Part model, mm, in its own coordinate system. Face numbers are marked on the shaded views. A direction names the side the tool comes from. Round coordinates to 2 decimals unless told otherwise and drop trailing zeros. Write each loop counter-clockwise with the first axis right and the second up, starting at its lowest first coordinate (ties: lowest second). Pieces come first, ordered by that corner, then holes.
1) Which spindle directions (+Z, -Z, +X, -X, +Y, -Y) get a long thin tool onto all of the face, cutting with end or side? Do the marked faces 4 and 5. Say none if no direction does.
2) Saw through at D-D on x = -68. Write the cut outline in (y, z), and give its area (3 significant figures).
3) Saw through at A-A on y = 5. Write the cut outline in (x, z).
4) Saw through at C-C on z = 138.5. Write the cut outline in (x, y).
5) Drill centre lines: L1, parallel to X at y = 45, z = 75; L2, parallel to X at y = 21.5, z = 96.5; L3, parallel to Y at x = -10, z = 5.2. Where is each one in solid material? Low to high.
6) Pull direction Y, two halves, no side cores. Call the marked faces 1, 2 and 3: +Y half, -Y half, draft (parallel to the pull), parting line (faces both ways), or undercut.
7) Flat gauge pins, fed straight in: pin 1 (5 mm diameter, centred on x = -165.5, z = 118.5, fed in from -Y); pin 2 (11 mm diameter, centred on x = -10.5, z = 93, fed in from -Y); pin 3 (4 mm diameter, centred on x = -10.5, y = 13, fed in from -Z). Where does each tip first touch, or does it go through?
8) Saw through at B-B on x = -10. Write the cut outline in (y, z).
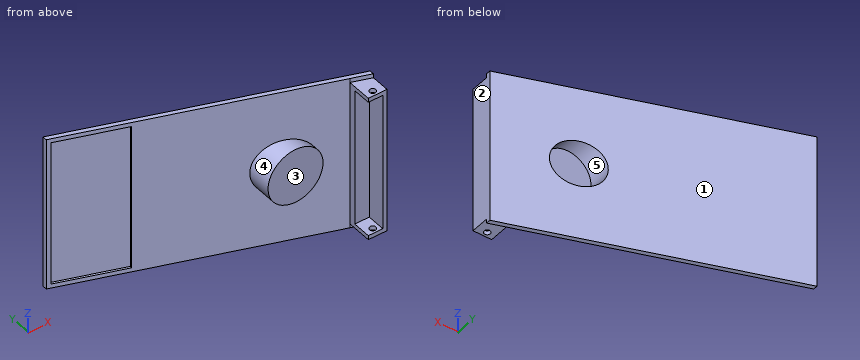
```python
from build123d import *

# Parameters (mm, degrees)
BOSS_EXTRUDE1_DEPTH = 150
CUT_EXTRUDE1_DEPTH  = 4
CUT_EXTRUDE2_DEPTH  = 4
SKETCH4_R           = 3
CUT_EXTRUDE3_DEPTH  = 162
SKETCH6_W           = 134
SKETCH6_H           = 17.5
CUT_EXTRUDE4_DEPTH  = 14
SKETCH9_R           = 22.5
CUT_EXTRUDE5_DEPTH  = 83
SKETCH10_R          = 26.5
BOSS_EXTRUDE2_DEPTH = 55
SKETCH12_R          = 26.5
CUT_EXTRUDE6_DEPTH  = 27
SKETCH13_R          = 22.5
CUT_EXTRUDE7_DEPTH  = 24
SKETCH14_W          = 65
SKETCH14_H          = 142
CUT_EXTRUDE8_DEPTH  = 2
SKETCH15_W          = 73.049040635
SKETCH15_H          = 56.643959476
CUT_EXTRUDE9_DEPTH  = 22


with BuildPart() as part:
    # Sketch1 → Boss-Extrude1 (new body)
    with BuildSketch(Plane.XY):
        Polygon((0, 0), (0, 21.74), (-249.999833435, 109.239715329), (-249.999833435, 104.999731628), (-18, 23.8), (-18, 0), align=None)
    extrude(amount=BOSS_EXTRUDE1_DEPTH)

    # Sketch2 → Cut-Extrude1 (cut)
    with BuildSketch(Plane.XY.offset(150)):
        Polygon((-18, 23.8), (0, 17.500016299), (0, 0), (-18, 0), align=None)
    extrude(amount=-CUT_EXTRUDE1_DEPTH, mode=Mode.SUBTRACT)

    # Sketch3 → Cut-Extrude2 (cut)
    with BuildSketch(Plane(origin=(0, 0, 0), x_dir=(-1, 0, 0), z_dir=(0, 0, -1))):
        Polygon((18, 0), (18, 23.8), (0, 17.500016299), (0, 0), align=None)
    extrude(amount=-CUT_EXTRUDE2_DEPTH, mode=Mode.SUBTRACT)

    # Sketch4 → Cut-Extrude3 (cut)
    with BuildSketch(Plane(origin=(0, 0, 4), x_dir=(-1, 0, 0), z_dir=(0, 0, -1))):
        with Locations((10, 5)):
            Circle(SKETCH4_R)
    extrude(amount=-CUT_EXTRUDE3_DEPTH, mode=Mode.SUBTRACT)

    # Sketch6 → Cut-Extrude4 (cut)
    with BuildSketch(Plane.ZY.offset(18)):
        with Locations((75, 8.75)):
            Rectangle(SKETCH6_W, SKETCH6_H)
    extrude(amount=-CUT_EXTRUDE4_DEPTH, mode=Mode.SUBTRACT)

    # Sketch9 → Cut-Extrude5 (cut)
    with BuildSketch(Plane(origin=(0, 0, 0), x_dir=(1, 0, 0), z_dir=(0, 1, 0))):
        with Locations((-68, -75)):
            Circle(SKETCH9_R)
    extrude(amount=CUT_EXTRUDE5_DEPTH, mode=Mode.SUBTRACT)

    # Sketch10 → Boss-Extrude2 (add)
    with BuildSketch(Plane(origin=(0, 0, 0), x_dir=(1, 0, 0), z_dir=(0, 1, 0))):
        with Locations((-68, -75)):
            Circle(SKETCH10_R)
    extrude(amount=BOSS_EXTRUDE2_DEPTH)

    # Sketch12 → Cut-Extrude6 (cut)
    with BuildSketch(Plane.XZ):
        with Locations(Location((-68, 75, 0), (0, 0, 270))):
            Circle(SKETCH12_R)
    extrude(amount=-CUT_EXTRUDE6_DEPTH, mode=Mode.SUBTRACT)

    # Sketch13 → Cut-Extrude7 (cut)
    with BuildSketch(Plane(origin=(0, 55, 0), x_dir=(1, 0, 0), z_dir=(0, 1, 0))):
        with Locations(Location((-68, -75, 0), (0, 0, 270))):
            Circle(SKETCH13_R)
    extrude(amount=-CUT_EXTRUDE7_DEPTH, mode=Mode.SUBTRACT)

    # Sketch14 → Cut-Extrude8 (cut)
    with BuildSketch(Plane(origin=(5.456564202, 15.590223769, 0), x_dir=(0.9438586228518121, -0.3303496633391366, 0), z_dir=(-0.3303496633391366, -0.9438586228518121, 0))):
        with Locations((-234.151124493, 75)):
            Rectangle(SKETCH14_W, SKETCH14_H)
    extrude(amount=-CUT_EXTRUDE8_DEPTH, mode=Mode.SUBTRACT)

    # Sketch15 → Cut-Extrude9 (cut)
    with BuildSketch(Plane(origin=(6.778605444, 19.367494233, 0), x_dir=(0.9438586228518122, -0.330349663339136, 0), z_dir=(0.330349663339136, 0.9438586228518122, 0))):
        with Locations((-76.286643032, -75.675013618)):
            Rectangle(SKETCH15_W, SKETCH15_H)
    extrude(amount=CUT_EXTRUDE9_DEPTH, mode=Mode.SUBTRACT)


solid = part.part
```
Completed:
1. face 4: -Y
1. face 5: +Y
2. outline: (27, 48.5) - (41.3, 48.5) - (41.3, 0) - (45.54, 0) - (45.54, 52.5) - (31, 52.5) - (31, 97.5) - (45.54, 97.5) - (45.54, 150) - (41.3, 150) - (41.3, 101.5) - (27, 101.5) - close
2. area: 740 mm2
3. outline: (-18, 4) - (-13, 4) - (-13, 8) - (-18, 8) - close; (-18, 142) - (-13, 142) - (-13, 146) - (-18, 146) - close; (-7, 4) - (0, 4) - (0, 146) - (-7, 146) - (-7, 142) - (-4, 142) - (-4, 8) - (-7, 8) - close
4. outline: (-250, 105) - (-246.22, 103.68) - (-245.56, 105.57) - (-184.21, 84.09) - (-184.87, 82.21) - (-18, 23.8) - (-18, 17.5) - (-4, 17.5) - (-4, 0) - (0, 0) - (0, 21.74) - (-250, 109.24) - close
5. L1: x = -94.5 to -90.5
5. L2: x = -18 to 0
5. L3: y = 0 to 2, 8 to 25.24
6. face 1: +Y half
6. face 2: draft
6. face 3: -Y half
7. pin 1: stops at y = 74.55
7. pin 2: stops at y = 17.5
7. pin 3: stops at z = 4
8. outline: (0, 4) - (2, 4) - (2, 8) - (0, 8) - close; (0, 142) - (2, 142) - (2, 146) - (0, 146) - close; (8, 4) - (21, 4) - (21, 0) - (25.24, 0) - (25.24, 150) - (21, 150) - (21, 146) - (8, 146) - (8, 142) - (17.5, 142) - (17.5, 8) - (8, 8) - close
